Could you check a few things on this drawing? It's one solid part, dimensions in mm from its lowest x, y, z. A direction names the side the tool comes from. Give positions to 0.01 mm unless a question says otherwise; leave off trailing zeros. Order: outer loops, then holes, each group sorted by start corner. A loop starts at its lowest first (then second) coordinate and runs counter-clockwise, first axis right, second up.
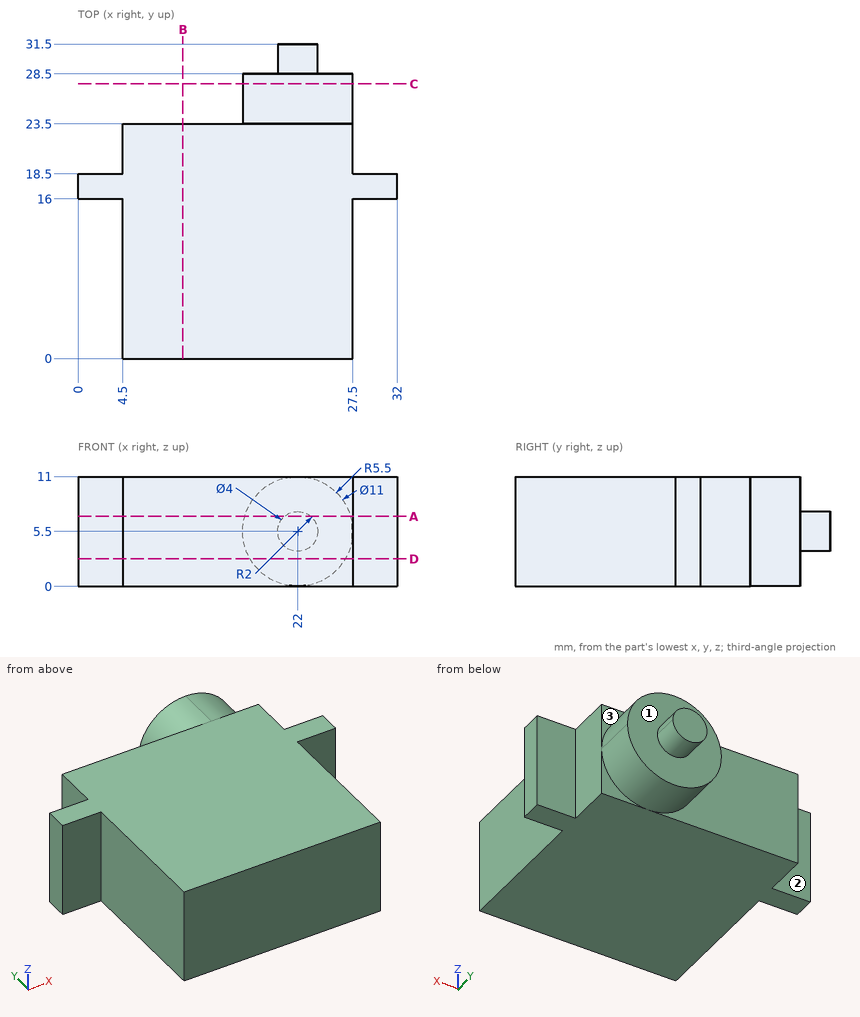
Item 1: For the marked faces 1, 2 and 3, which set-ups out of +Z, -Z, +X, -X, +Y, -Y let a thin tool reach every point of the face, with its end or its side?
Findings:
face 1: +Y
face 2: +Z, -Z, -X, +Y
face 3: +Z, +X, +Y
Item 2: Imagine slicing it at B-B on x = 10.5. List the corners of the cut face in (y, z) for me, then the cut area to 4 significant figures.
Findings:
outline: (0, 0) - (23.5, 0) - (23.5, 11) - (0, 11) - close
area: 258.5 mm2
Item 3: For pin 1 (5.5 mm diameter, centred on y = 6.5, z = 6.5, fed in from +X); pin 2 (1 mm diameter, centred on x = 17, y = 27, fed in from -Z); pin 3 (3.5 mm diameter, centred on x = 29.5, z = 4, fed in from -Y), each with a flat end and sliding along its axis, tell me the tip position at first contact or that it passes through.
Findings:
pin 1: stops at x = 27.5
pin 2: stops at z = 2.34
pin 3: stops at y = 16
Item 4: Please list where these lines run through material, in increasing order: line 1 along Y through (x, z) = (24, 3.5); line 2 along Y through (x, z) = (5.5, 5.5); line 3 along X through (y, z) = (11, 4.25).
Findings:
line 1: y = 0 to 28.5
line 2: y = 0 to 23.5
line 3: x = 4.5 to 27.5
Item 5: Imagine slicing it at A-A on z = 7. List the corners of the cut face in (x, y) for me.
Findings:
outline: (0, 16) - (4.5, 16) - (4.5, 0) - (27.5, 0) - (27.5, 16) - (32, 16) - (32, 18.5) - (27.5, 18.5) - (27.5, 23.5) - (27.29, 23.5) - (27.29, 28.5) - (23.32, 28.5) - (23.32, 31.5) - (20.68, 31.5) - (20.68, 28.5) - (16.71, 28.5) - (16.71, 23.5) - (4.5, 23.5) - (4.5, 18.5) - (0, 18.5) - close
Item 6: Imagine slicing it at D-D on z = 2.75. List the corners of the cut face in (x, y) for me.
Findings:
outline: (0, 16) - (4.5, 16) - (4.5, 0) - (27.5, 0) - (27.5, 16) - (32, 16) - (32, 18.5) - (27.5, 18.5) - (27.5, 23.5) - (26.76, 23.5) - (26.76, 28.5) - (17.24, 28.5) - (17.24, 23.5) - (4.5, 23.5) - (4.5, 18.5) - (0, 18.5) - close
Item 7: Imagine slicing it at C-C on y = 27.5. List the corners of the cut face in (x, z) for me.
Findings:
outline: circle Ø11 at (22, 5.5)
